The listing builds one solid part. Answer for the finished solid, in the listing's coordinates (mm). Face numbers are marked on the shaded views. A direction names the side the tool comes from. Round coordinates to 2 decimals unless told otherwise and drop trailing zeros. Write each loop counter-clockwise with the first axis right and the second up, starting at its lowest first coordinate (ties: lowest second). Pieces come first, ordered by that corner, then holes. Notation, with made-up numbers: M -13.75,2 L -0.75,2 A38 cw -0.75,40 Z; hole C 26.5,84 d9. An arc over 180 degrees is marked long. Write each question's results on one line, items separated by ' | '.
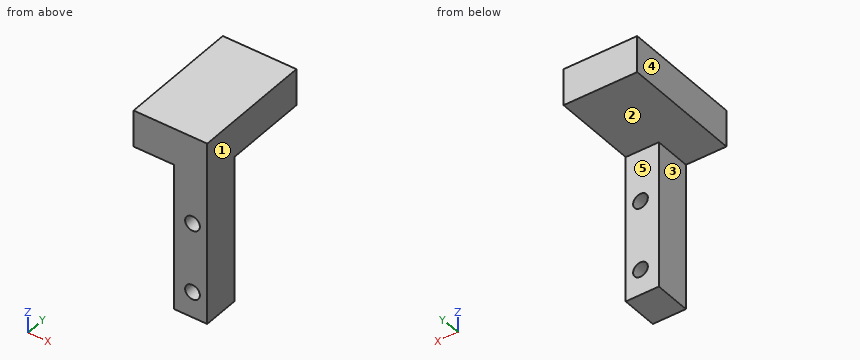
from build123d import *

# Parameters (mm, degrees)
SKETCH1_W           = 10
SKETCH1_H           = 10
BOSS_EXTRUDE1_DEPTH = 50
SKETCH3_W           = 10
SKETCH3_H           = 10
BOSS_EXTRUDE3_DEPTH = 11
SKETCH8_W           = 20
SKETCH8_H           = 10
BOSS_EXTRUDE4_DEPTH = 23
SKETCH9_R           = 2
CUT_EXTRUDE2_DEPTH  = 23
SKETCH9_4_R         = 2
CUT_EXTRUDE3_DEPTH  = 23
SKETCH_1_W          = 50
SKETCH_1_H          = 10
CUT_EXTRUDE_1_DEPTH = 1


with BuildPart() as part:
    # Sketch1 → Boss-Extrude1 (new body)
    with BuildSketch(Plane.XY):
        with Locations((-2.851282988, -1.356707317)):
            Rectangle(SKETCH1_W, SKETCH1_H)
    extrude(amount=BOSS_EXTRUDE1_DEPTH)

    # Sketch3 → Boss-Extrude3 (add)
    with BuildSketch(Plane.ZY.offset(7.851282988)):
        with Locations((45, -1.356707317)):
            Rectangle(SKETCH3_W, SKETCH3_H)
    extrude(amount=BOSS_EXTRUDE3_DEPTH)

    # Sketch8 → Boss-Extrude4 (add)
    with BuildSketch(Plane(origin=(0, 3.643292683, 0), x_dir=(1, 0, 0), z_dir=(0, 1, 0))):
        with Locations((-8.851282988, -45)):
            Rectangle(SKETCH8_W, SKETCH8_H)
    extrude(amount=BOSS_EXTRUDE4_DEPTH)

    # Sketch9 → Cut-Extrude2 (cut)
    with BuildSketch(Plane(origin=(0, 3.643292683, 0), x_dir=(1, 0, 0), z_dir=(0, 1, 0))):
        with Locations(Location((-2.851282988, -7, 0), (0, 0, 270))):
            Circle(SKETCH9_R)
    extrude(amount=-CUT_EXTRUDE2_DEPTH, mode=Mode.SUBTRACT)

    # Sketch9<4> → Cut-Extrude3 (cut)
    with BuildSketch(Plane(origin=(0, 3.643292683, 0), x_dir=(1, 0, 0), z_dir=(0, 1, 0))):
        with Locations(Location((-2.851282988, -26, 0), (0, 0, 270))):
            Circle(SKETCH9_4_R)
    extrude(amount=-CUT_EXTRUDE3_DEPTH, mode=Mode.SUBTRACT)

    # 草图1 → 切除-拉伸1 (cut)
    with BuildSketch(Plane(origin=(2.148717012, 0, 0), x_dir=(0, 0, -1), z_dir=(1, 0, 0))):
        with Locations((-25, -1.356707317)):
            Rectangle(SKETCH_1_W, SKETCH_1_H)
    extrude(amount=-CUT_EXTRUDE_1_DEPTH, mode=Mode.SUBTRACT)


solid = part.part
1) A tool of negligible diameter and unlimited length cuts with its end or side. For the marked faces 1, 2, 3, 4 and 5, from which of +Z, -Z, +X, -X, +Y, -Y can it reach the whole face along a straight path? Write none if from no direction.
Return value:
face 1: +Z, -Z, +X, +Y, -Y | face 2: -Z, -X, +Y | face 3: -Z, -X, +Y, -Y | face 4: +Z, -Z, -X, +Y, -Y | face 5: -Z, +X, -X, +Y
2) Each of these flat-tipped pins is pushed along its axis until it touches: pin 1 (3 mm diameter, centred on y = -0.5, z = 22, fed in from -X); pin 2 (12 mm diameter, centred on x = -17, z = 37, fed in from -Y); pin 3 (6.5 mm diameter, centred on x = -2.85, z = 7, fed in from +Y); pin 4 (10 mm diameter, centred on x = -12.5, y = 13.5, fed in from -Z). Where does it stop, or does it pass through?
Return value:
pin 1: x = -7.85 | pin 2: y = -6.36 | pin 3: y = 3.64 | pin 4: z = 40
3) Section A-A (z = 7) is taken. Determine the outline of the cut face in (x, y).
Return value:
outline: M -7.85,-6.36 L -4.85,-6.36 L -4.85,3.64 L -7.85,3.64 Z; M -0.85,-6.36 L 1.15,-6.36 L 1.15,3.64 L -0.85,3.64 Z
4) Section D-D (y = 14.5) is taken. Determine the outline of the cut face in (x, z).
Return value:
outline: M -18.85,40 L 1.15,40 L 1.15,50 L -18.85,50 Z
5) Find the intervals of material crossed by line 1 (X direction, y = -1.75, z = 7); line 2 (Z direction, x = -3.5, y = -0.5); line 3 (Z direction, x = -16.25, y = 7), in increasing order.
Return value:
line 1: -7.85 to -4.85, -0.85 to 1.15 | line 2: 0 to 5.11, 8.89 to 24.11, 27.89 to 50 | line 3: 40 to 50
6) Section B-B (y = 1) is taken. Determine the outline of the cut face in (x, z), then the cut area to 3 significant figures.
Return value:
outline: M -18.85,40 L -7.85,40 L -7.85,0 L 1.15,0 L 1.15,50 L -18.85,50 Z; hole C -2.85,7 d4; hole C -2.85,26 d4 | area: 535 mm²
7) Section C-C (x = -15.5) is taken. Determine the outline of the cut face in (y, z).
Return value:
outline: M -6.36,40 L 26.64,40 L 26.64,50 L -6.36,50 Z
